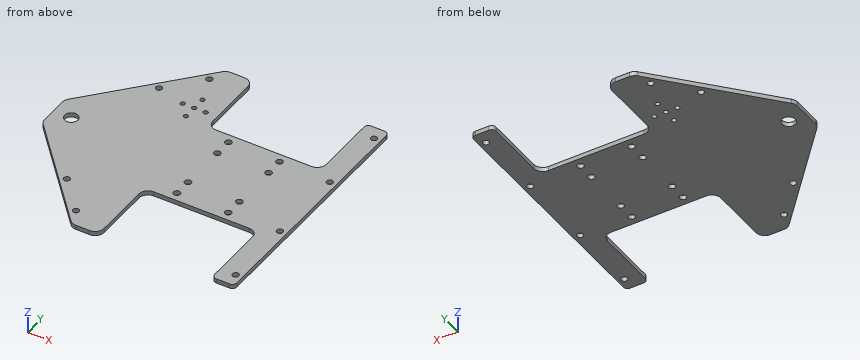
from build123d import *

# Parameters (mm, degrees)
SKETCH_R        = 2.3622
SKETCH_R_2      = 4.7625
PAD_DEPTH       = 3.175
FILLET_R        = 6.35
FILLET001_R     = 6.35
FILLET002_R     = 6.35
FILLET003_R     = 6.35
FILLET004_R     = 6.35
FILLET005_R     = 3.175
FILLET006_R     = 3.175
FILLET007_R     = 6.35
FILLET008_R     = 6.35
FILLET009_R     = 6.35
FILLET010_R     = 6.35
FILLET011_R     = 6.35
FILLET012_R     = 3.175
FILLET013_R     = 3.175
SKETCH001_R     = 1.651
POCKET_DEPTH    = 3.176
SKETCH002_R     = 2.2479
POCKET001_DEPTH = 3.176
SKETCH003_R     = 2.2479
POCKET002_DEPTH = 4.99999


with BuildPart() as part:
    # Sketch → Pad (new body)
    with BuildSketch(Plane(origin=(-14.3421, 44.2432, 43.6758), x_dir=(1, 0, 0), z_dir=(0, 0, 1))):
        Polygon((40.4368, 35.9029), (-40.4368, 35.9029), (-40.4368, 88.9), (-59.4868, 88.9), (-127.8382, 12.7), (-127.8382, -12.7), (-59.4868, -88.9), (-40.4368, -88.9), (-40.4368, -35.9029), (40.4368, -35.9029), (40.4368, -88.9), (56.3118, -88.9), (56.3118, 88.9), (40.4368, 88.9), align=None)
        with Locations((-21.3868, 29.5529)):
            Circle(SKETCH_R, mode=Mode.SUBTRACT)
        with Locations((-21.3868, 16.8529)):
            Circle(SKETCH_R, mode=Mode.SUBTRACT)
        with Locations((-21.3868, -16.8529)):
            Circle(SKETCH_R, mode=Mode.SUBTRACT)
        with Locations((-21.3868, -29.5529)):
            Circle(SKETCH_R, mode=Mode.SUBTRACT)
        with Locations((15.0368, 29.5529)):
            Circle(SKETCH_R, mode=Mode.SUBTRACT)
        with Locations((15.24, 16.8529)):
            Circle(SKETCH_R, mode=Mode.SUBTRACT)
        with Locations((15.24, -16.8529)):
            Circle(SKETCH_R, mode=Mode.SUBTRACT)
        with Locations((15.24, -29.5529)):
            Circle(SKETCH_R, mode=Mode.SUBTRACT)
        with Locations((-115.1382, 0)):
            Circle(SKETCH_R_2, mode=Mode.SUBTRACT)
    extrude(amount=PAD_DEPTH)

    # Fillet
    fillet_edges = [part.edges().sort_by_distance(p)[0] for p in [
        (-142.1803, 31.5432, 45.2633),
    ]]
    fillet(fillet_edges, radius=FILLET_R)

    # Fillet001
    fillet001_edges = [part.edges().sort_by_distance(p)[0] for p in [
        (-73.8289, -44.6568, 45.2633),
    ]]
    fillet(fillet001_edges, radius=FILLET001_R)

    # Fillet002
    fillet002_edges = [part.edges().sort_by_distance(p)[0] for p in [
        (-54.7789, -44.6568, 45.2633),
    ]]
    fillet(fillet002_edges, radius=FILLET002_R)

    # Fillet003
    fillet003_edges = [part.edges().sort_by_distance(p)[0] for p in [
        (-54.7789, 8.3403, 45.2633),
    ]]
    fillet(fillet003_edges, radius=FILLET003_R)

    # Fillet004
    fillet004_edges = [part.edges().sort_by_distance(p)[0] for p in [
        (26.0947, 8.3403, 45.2633),
    ]]
    fillet(fillet004_edges, radius=FILLET004_R)

    # Fillet005
    fillet005_edges = [part.edges().sort_by_distance(p)[0] for p in [
        (26.0947, -44.6568, 45.2633),
    ]]
    fillet(fillet005_edges, radius=FILLET005_R)

    # Fillet006
    fillet006_edges = [part.edges().sort_by_distance(p)[0] for p in [
        (41.9697, -44.6568, 45.2633),
    ]]
    fillet(fillet006_edges, radius=FILLET006_R)

    # Fillet007
    fillet007_edges = [part.edges().sort_by_distance(p)[0] for p in [
        (-142.1803, 56.9432, 45.2633),
    ]]
    fillet(fillet007_edges, radius=FILLET007_R)

    # Fillet008
    fillet008_edges = [part.edges().sort_by_distance(p)[0] for p in [
        (-73.8289, 133.1432, 45.2633),
    ]]
    fillet(fillet008_edges, radius=FILLET008_R)

    # Fillet009
    fillet009_edges = [part.edges().sort_by_distance(p)[0] for p in [
        (-54.7789, 133.1432, 45.2633),
    ]]
    fillet(fillet009_edges, radius=FILLET009_R)

    # Fillet010
    fillet010_edges = [part.edges().sort_by_distance(p)[0] for p in [
        (26.0947, 80.1461, 45.2633),
    ]]
    fillet(fillet010_edges, radius=FILLET010_R)

    # Fillet011
    fillet011_edges = [part.edges().sort_by_distance(p)[0] for p in [
        (-54.7789, 80.1461, 45.2633),
    ]]
    fillet(fillet011_edges, radius=FILLET011_R)

    # Fillet012
    fillet012_edges = [part.edges().sort_by_distance(p)[0] for p in [
        (26.0947, 133.1432, 45.2633),
    ]]
    fillet(fillet012_edges, radius=FILLET012_R)

    # Fillet013
    fillet013_edges = [part.edges().sort_by_distance(p)[0] for p in [
        (41.9697, 133.1432, 45.2633),
    ]]
    fillet(fillet013_edges, radius=FILLET013_R)

    # Sketch001 → Pocket (cut, through all)
    with BuildSketch(Plane(origin=(-14.3421, 44.2432, 46.8508), x_dir=(1, 0, 0), z_dir=(0, 0, 1))):
        with Locations((-56.906653, 47.390231)):
            Circle(SKETCH001_R)
        with Locations((-65.098153, 47.390231)):
            Circle(SKETCH001_R)
        with Locations((-56.906653, 56.915231)):
            Circle(SKETCH001_R)
        with Locations((-48.715153, 47.390231)):
            Circle(SKETCH001_R)
        with Locations((-56.906653, 37.865231)):
            Circle(SKETCH001_R)
    extrude(amount=-POCKET_DEPTH, mode=Mode.SUBTRACT)

    # Sketch002 → Pocket001 (cut, through all)
    with BuildSketch(Plane(origin=(-14.3421, 44.2432, 46.8508), x_dir=(1, 0, 0), z_dir=(0, 0, 1))):
        with Locations((-85.394727, -52.884764)):
            Circle(SKETCH002_R)
        with Locations((-64.1943, -76.519577)):
            Circle(SKETCH002_R)
        with Locations((-64.1943, 76.519577)):
            Circle(SKETCH002_R)
        with Locations((-85.394727, 52.884764)):
            Circle(SKETCH002_R)
    extrude(amount=-POCKET001_DEPTH, mode=Mode.SUBTRACT)

    # Sketch003 → Pocket002 (cut)
    with BuildSketch(Plane(origin=(-14.3421, 44.2432, 46.8508), x_dir=(1, 0, 0), z_dir=(0, 0, 1))):
        with Locations((51.5493, -79.375)):
            Circle(SKETCH003_R)
        with Locations((51.5493, -28.575)):
            Circle(SKETCH003_R)
        with Locations((51.5493, 79.375)):
            Circle(SKETCH003_R)
        with Locations((51.5493, 28.575)):
            Circle(SKETCH003_R)
    extrude(amount=-POCKET002_DEPTH, mode=Mode.SUBTRACT)


solid = part.part
Can you work these out from the model? Positions are in its coordinate system, mm. Coordinates: 2 decimals unless noted, no trailing zeros. Write each loop counter-clockwise with the first axis right and the second up, starting at its lowest first coordinate (ties: lowest second). Pieces come first, ordered by that corner, then holes. Notation, with made-up numbers: (48.25, 77) -> (103.25, 77) arc R31 cw to (103.25, 108) -> close; hole circle Ø7 at (33.5, 29). An arc over 180 degrees is marked (long way). Write each question's results on one line, items separated by ' | '. Start each with the question number.
Item 1: Please list where these lines run through material, in increasing order: probe 1 along X at (y, z) = (-10, 45.45); probe 2 along Y at (x, z) = (-99.5, 44.9); probe 3 along X at (y, z) = (25.5, 43.8).
Item 2: If we section it at B-B, the plane x = -30.5: Write out the boundary of the cut face in (y, z), and give its area (3 significant figures).
Item 3: If we section it at C-C, the plane y = 113.5: Write out the boundary of the cut face in (x, z).
Item 4: I'm going to push flat-ended pins straight in: P1, Ø6, axis at x = -35.73, y = 27.39, coming from the +Z side; P2, Ø1, axis at x = -13, z = 45, coming from the +Y side. Where does each tip first touch, or does it pass through?
Item 5: If we section it at A-A, the plane y = 6: Write out the boundary of the cut face in (x, z).
Item 6: If we section it at D-D, the plane z = 45.8: Count the separate pieces of the cut face and the enclosed holes in it, and give its area (3 significant figures).
Answer block:
1) probe 1: -104.92 to -101.53, -97.95 to -54.78, 26.09 to 41.97 | probe 2: -16.04 to -10.88, -6.41 to 94.89, 99.36 to 104.52 | probe 3: -136.76 to -37.15, -34.31 to -0.52, 2.31 to 41.97
2) outline: (8.34, 43.68) -> (80.15, 43.68) -> (80.15, 46.85) -> (8.34, 46.85) -> close | area: 228 mm²
3) outline: (-91.45, 43.68) -> (-54.78, 43.68) -> (-54.78, 46.85) -> (-91.45, 46.85) -> close; (26.09, 43.68) -> (41.97, 43.68) -> (41.97, 46.85) -> (26.09, 46.85) -> close
4) P1: z = 46.85 | P2: y = 80.15
5) outline: (-119.27, 43.68) -> (-53.35, 43.68) -> (-53.35, 46.85) -> (-119.27, 46.85) -> close; (24.67, 43.68) -> (41.97, 43.68) -> (41.97, 46.85) -> (24.67, 46.85) -> close
6) separate pieces: 1 | enclosed holes: 22 | area: 18,600 mm²
